Work out the finished part from the listing and answer in its coordinate system (mm). Coordinates: 2 decimals unless noted, no trailing zeros. Loops run counter-clockwise (first coordinate to the right, second up) from the corner with the lowest first, then second, coordinate; pieces in that order, holes last.
```python
from build123d import *
from OCP.BRepFilletAPI import BRepFilletAPI_MakeChamfer

# Parameters (mm, degrees)
SZKIC1_R                    = 6
DODANIE_WYCI_GNI_CIE1_DEPTH = 10.8
SZKIC2_OUTSIDE_W            = 89.934
SZKIC2_OUTSIDE_H            = 92.718
SZKIC2_OUTSIDE_R            = 8.3
WYTNIJ_WYCI_GNI_CIE1_DEPTH  = 18.482562741
WYTNIJ_WYCI_GNI_CIE1_DRAFT  = -60
SZKIC3_OUTSIDE_W            = 89.934
SZKIC3_OUTSIDE_H            = 92.718
SZKIC3_OUTSIDE_R            = 8.3
WYTNIJ_WYCI_GNI_CIE3_DEPTH  = 18.482562741
WYTNIJ_WYCI_GNI_CIE3_DRAFT  = -60
SFAZOWANIE2_SIZE            = 0.5
SFAZOWANIE2_SIZE2           = 0.288675135


with BuildPart() as part:
    # Szkic1 → Dodanie-wyciągnięcie1 (new body)
    with BuildSketch(Plane.XY):
        Polygon((0, 10.392304845), (-9, 5.196152423), (-9, -5.196152423), (0, -10.392304845), (9, -5.196152423), (9, 5.196152423), align=None)
        with Locations(Location((0, 0, 0), (0, 0, 180))):
            Circle(SZKIC1_R, mode=Mode.SUBTRACT)
    extrude(amount=DODANIE_WYCI_GNI_CIE1_DEPTH)


with BuildPart() as wytnij_wyci_gni_cie1_tool:
    # Szkic2 outside → Wytnij-wyciągnięcie1 (with draft: the straight prism first)
    with BuildSketch(Plane.XY.offset(10.8)):
        Rectangle(SZKIC2_OUTSIDE_W, SZKIC2_OUTSIDE_H)
        Circle(SZKIC2_OUTSIDE_R, mode=Mode.SUBTRACT)
    extrude(amount=-WYTNIJ_WYCI_GNI_CIE1_DEPTH)
    # Wytnij-wyciągnięcie1: the draft: its side faces are tilted about the plane it starts from
    wytnij_wyci_gni_cie1_sides = [wytnij_wyci_gni_cie1_tool.faces().sort_by_distance(p)[0] for p in [
        (0, -46.359, 1.558718629),
        (44.967, 0, 1.558718629),
        (0, 46.359, 1.558718629),
        (-44.967, 0, 1.558718629),
        (-8.3, 0, 1.558718629),
    ]]
    draft(wytnij_wyci_gni_cie1_sides, Plane.XY.offset(10.8), WYTNIJ_WYCI_GNI_CIE1_DRAFT)


with BuildPart() as part_1:
    add(part.part)

    # Wytnij-wyciągnięcie1: cut by wytnij_wyci_gni_cie1_tool
    add(wytnij_wyci_gni_cie1_tool.part, mode=Mode.SUBTRACT)


with BuildPart() as wytnij_wyci_gni_cie3_tool:
    # Szkic3 outside → Wytnij-wyciągnięcie3 (with draft: the straight prism first)
    with BuildSketch(Plane(origin=(0, 0, 0), x_dir=(-1, 0, 0), z_dir=(0, 0, -1))):
        Rectangle(SZKIC3_OUTSIDE_W, SZKIC3_OUTSIDE_H)
        Circle(SZKIC3_OUTSIDE_R, mode=Mode.SUBTRACT)
    extrude(amount=-WYTNIJ_WYCI_GNI_CIE3_DEPTH)
    # Wytnij-wyciągnięcie3: the draft: its side faces are tilted about the plane it starts from
    wytnij_wyci_gni_cie3_sides = [wytnij_wyci_gni_cie3_tool.faces().sort_by_distance(p)[0] for p in [
        (0, -46.359, 9.241281371),
        (-44.967, 0, 9.241281371),
        (0, 46.359, 9.241281371),
        (44.967, 0, 9.241281371),
        (8.3, 0, 9.241281371),
    ]]
    draft(wytnij_wyci_gni_cie3_sides, Plane(origin=(0, 0, 0), x_dir=(-1, 0, 0), z_dir=(0, 0, -1)), WYTNIJ_WYCI_GNI_CIE3_DRAFT)


with BuildPart() as part_2:
    add(part_1.part)

    # Wytnij-wyciągnięcie3: cut by wytnij_wyci_gni_cie3_tool
    add(wytnij_wyci_gni_cie3_tool.part, mode=Mode.SUBTRACT)

    # Sfazowanie2: one chamfer whose edges measure the first distance from different faces: ONE call of the kernel's chamfer builder (chamfer() names one face for all edges)
    sfazowanie2_edges_1 = [part_2.edges().sort_by_distance(p)[0] for p in [
        (6, 0, 0),
    ]]
    sfazowanie2_side_1 = [part_2.faces().sort_by_distance(p)[0] for p in [
        (6, 0, 5.4),
    ]]
    sfazowanie2_edges_2 = [part_2.edges().sort_by_distance(p)[0] for p in [
        (6, 0, 10.8),
    ]]
    sfazowanie2_side_2 = [part_2.faces().sort_by_distance(p)[0] for p in [
        (-8.065240549, 0, 10.8),
    ]]
    sfazowanie2 = BRepFilletAPI_MakeChamfer(part_2.part.solid().wrapped)
    for e in sfazowanie2_edges_1:
        sfazowanie2.Add(SFAZOWANIE2_SIZE, SFAZOWANIE2_SIZE2, e.wrapped, sfazowanie2_side_1[0].wrapped)  # the first distance lies on this face
    for e in sfazowanie2_edges_2:
        sfazowanie2.Add(SFAZOWANIE2_SIZE, SFAZOWANIE2_SIZE2, e.wrapped, sfazowanie2_side_2[0].wrapped)  # the first distance lies on this face
    add(Compound.cast(sfazowanie2.Shape()), mode=Mode.REPLACE)


solid = part_2.part
```
1. A cutting plane is placed at B-B, the plane z = 1.5. Give the vertices of the cut face in (x, y).
2. Each of these flat-tipped pins is pushed along its axis until it touches: P1, Ø4, axis at x = 2.5, z = 3, coming from the +Y side; P2, Ø1, axis at y = 7, z = 4.5, coming from the +X side; P3, Ø4, axis at x = -6.5, z = 8.5, coming from the -Y side. Where does it stop, or does it pass through?
3. Straight lines are drawn through the part: probe 1 along Y at (x, z) = (-6.75, 1); probe 2 along Y at (x, z) = (4.75, 2.5); probe 3 along X at (y, z) = (-4.5, 6.5). For each, find the intervals that lie inside material, in ascending order.
4. Determine the mould class of faces 1 (the flat face through (-4.56, -7.76, 5.33)), 2 (the cylindrical face through (-5.723, -1.802, 5.436)), 3 (the flat face through (-4.44, 7.83, 5.33)), 4 (the flat face through (9, 0, 5)) for opening direction Y: released by +Y, released by -Y, zero draft, split by the parting line, or undercut.
5. A cutting plane is placed at A-A, the plane y = 0. Give the vertices of the cut face in (x, z), then the cut area to 3 significant figures.
Answers below:
1. outline: (-9, -5.2) - (0, -10.39) - (9, -5.2) - (9, 5.2) - (0, 10.39) - (-9, 5.2) - close; hole circle Ø12 at (0, 0)
2. P1: stops at y = 10.1
2. P2: stops at x = 6.74
2. P3: stops at y = -7.79
3. probe 1: y = -6.5 to 6.5
3. probe 2: y = -7.65 to -3.67, 3.67 to 7.65
3. probe 3: x = -9 to -3.97, 3.97 to 9
4. face 1: released by -Y
4. face 2: undercut
4. face 3: released by +Y
4. face 4: zero draft
5. outline: (-9, 0.4) - (-8.3, 0) - (-6.29, 0) - (-6, 0.5) - (-6, 10.51) - (-6.5, 10.8) - (-8.3, 10.8) - (-9, 10.4) - close; (6, 0.5) - (6.29, 0) - (8.3, 0) - (9, 0.4) - (9, 10.4) - (8.3, 10.8) - (6.5, 10.8) - (6, 10.51) - close
5. area: 63.9 mm2
